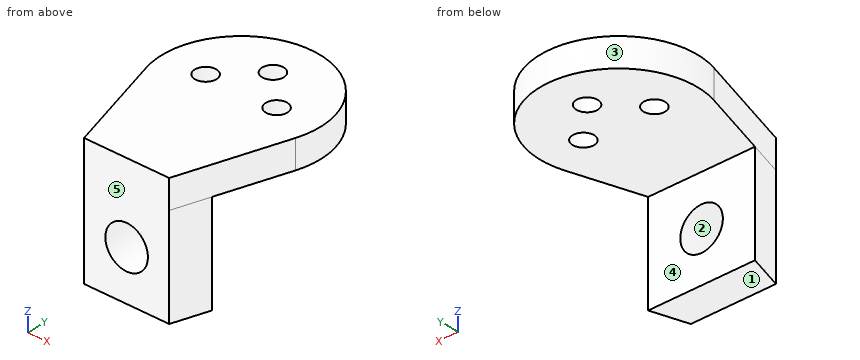
```python
from build123d import *

# Parameters (mm, degrees)
SKETCH1_R           = 55
BOSS_EXTRUDE1_DEPTH = 20
BOSS_EXTRUDE2_DEPTH = 20
CUT_EXTRUDE2_REACH  = 22
SKETCH4_R           = 7.5
BOSS_EXTRUDE3_DEPTH = 70
CUT_EXTRUDE3_REACH  = 27
SKETCH6_R           = 15


with BuildPart() as part:
    # Sketch1 → Boss-Extrude1 (new body)
    with BuildSketch(Plane.XY):
        Circle(SKETCH1_R)
    extrude(amount=BOSS_EXTRUDE1_DEPTH)

    # Sketch2 → Boss-Extrude2 (add)
    with BuildSketch(Plane.XY.offset(20)):
        with BuildLine():
            ThreePointArc((52.597301626, -16.078677236), (0, -55), (-52.597301626, -16.078677236))
            Line((-52.597301626, -16.078677236), (-30, -90))
            Line((-30, -90), (30, -90))
            Line((30, -90), (52.597301626, -16.078677236))
        make_face()
    extrude(amount=-BOSS_EXTRUDE2_DEPTH)

    # Sketch4 → Cut-Extrude2 (cut, up to next)
    with BuildSketch(Plane(origin=(0, 0, 0), x_dir=(-1, 0, 0), z_dir=(0, 0, -1)), mode=Mode.PRIVATE) as cut_extrude2_sk1:
        with Locations((0, 25)):
            Circle(SKETCH4_R)
    cut_extrude2_tool1 = extrude(cut_extrude2_sk1.sketch, amount=-CUT_EXTRUDE2_REACH, mode=Mode.PRIVATE) & part.part
    add(cut_extrude2_tool1.solids().sort_by_distance((0, 25, 0))[0], mode=Mode.SUBTRACT)
    # Sketch4 → Cut-Extrude2 (cut, up to next)
    with BuildSketch(Plane(origin=(0, 0, 0), x_dir=(-1, 0, 0), z_dir=(0, 0, -1)), mode=Mode.PRIVATE) as cut_extrude2_sk2:
        with Locations((-25, 0)):
            Circle(SKETCH4_R)
    cut_extrude2_tool2 = extrude(cut_extrude2_sk2.sketch, amount=-CUT_EXTRUDE2_REACH, mode=Mode.PRIVATE) & part.part
    add(cut_extrude2_tool2.solids().sort_by_distance((25, 0, 0))[0], mode=Mode.SUBTRACT)
    # Sketch4 → Cut-Extrude2 (cut, up to next)
    with BuildSketch(Plane(origin=(0, 0, 0), x_dir=(-1, 0, 0), z_dir=(0, 0, -1)), mode=Mode.PRIVATE) as cut_extrude2_sk3:
        with Locations((25, 0)):
            Circle(SKETCH4_R)
    cut_extrude2_tool3 = extrude(cut_extrude2_sk3.sketch, amount=-CUT_EXTRUDE2_REACH, mode=Mode.PRIVATE) & part.part
    add(cut_extrude2_tool3.solids().sort_by_distance((-25, 0, 0))[0], mode=Mode.SUBTRACT)

    # Sketch5 → Boss-Extrude3 (add)
    with BuildSketch(Plane(origin=(0, 0, 0), x_dir=(-1, 0, 0), z_dir=(0, 0, -1))):
        Polygon((37.642348913, -65), (-37.642348913, -65), (-30, -90), (30, -90), align=None)
    extrude(amount=BOSS_EXTRUDE3_DEPTH)

    # Sketch6 → Cut-Extrude3 (cut, up to next)
    with BuildSketch(Plane(origin=(0, -65, 0), x_dir=(1, 0, 0), z_dir=(0, 1, 0)), mode=Mode.PRIVATE) as cut_extrude3_sk1:
        with Locations((0, 35)):
            Circle(SKETCH6_R)
    cut_extrude3_tool1 = extrude(cut_extrude3_sk1.sketch, amount=-CUT_EXTRUDE3_REACH, mode=Mode.PRIVATE) & part.part
    add(cut_extrude3_tool1.solids().sort_by_distance((0, -65, -35))[0], mode=Mode.SUBTRACT)


solid = part.part
```
CAD build for the part. Positions are in the model's coordinates, mm. Face numbers are marked on the shaded views. A direction names the side the tool comes from. Coordinates: 2 decimals unless noted, no trailing zeros. Order: outer loops, then holes, each group sorted by start corner. A loop starts at its lowest first (then second) coordinate and runs counter-clockwise, first axis right, second up. Notation, with made-up numbers: M 83.5,39.5 L 140.5,39.5 A34 cw 140.5,73.5 Z; hole C 12,21 d2. An arc over 180 degrees is marked long. Answer as CSV lines item,"result".
1) Cut at C-C (x = 0). List the corners of the cut face in (y, z).
Verdict:
outline,"M -90,-70 L -65,-70 L -65,-50 L -90,-50 Z; M -90,-20 L -65,-20 L -65,0 L 17.5,0 L 17.5,20 L -90,20 Z; M 32.5,0 L 55,0 L 55,20 L 32.5,20 Z"
2) Cut at D-D (y = 25). List the corners of the cut face in (x, z).
Verdict:
outline,"M -48.99,0 L -7.5,0 L -7.5,20 L -48.99,20 Z; M 7.5,0 L 48.99,0 L 48.99,20 L 7.5,20 Z"
3) Drill centre lines: L1, parallel to Z at x = 0, y = -72.75; L2, parallel to Z at x = -36, y = 29.5; L3, parallel to Y at x = -29, z = -20.5. Where is each one in solid material? Low to high. Write a range as from..to.
Verdict:
L1,"-70..-50, -20..20"
L2,"0..20"
L3,"-90..-65"
4) Cut at A-A (y = 0). List the corners of the cut face in (x, z).
Verdict:
outline,"M -55,0 L -32.5,0 L -32.5,20 L -55,20 Z; M -17.5,0 L 17.5,0 L 17.5,20 L -17.5,20 Z; M 32.5,0 L 55,0 L 55,20 L 32.5,20 Z"
5) Flat gauge pins, fed straight in: P1, Ø12, axis at x = -25, y = 0, coming from the -Z side; P2, Ø10, axis at x = -42.5, z = -44, coming from the +Y side; P3, Ø17, axis at x = 25, y = 0, coming from the +Z side; P4, Ø17, axis at x = 0, y = 25, coming from the -Z side. Where does each tip first touch, or does it go through?
Verdict:
P1,"through"
P2,"y = -65"
P3,"z = 20"
P4,"z = 0"
6) Mould opens along Z. For the marked faces 1, 2 and 3 say: released by +Z, released by -Z, zero draft, split by the parting line, or undercut.
Verdict:
face 1,"released by -Z"
face 2,"undercut"
face 3,"zero draft"
7) Cut at B-B (z = -35). List the corners of the cut face in (x, y).
Verdict:
outline,"M -37.64,-65 L -30,-90 L -15,-90 L -15,-65 Z; M 15,-90 L 30,-90 L 37.64,-65 L 15,-65 Z"
8) 3-axis set-ups, long thin cutter, end or side, ignore diameter. For the marked faces 4 and 5: which of +Z, -Z, +X, -X, +Y, -Y reach the whole face in a straight line?
Verdict:
face 4,"-Z, +X, -X, +Y"
face 5,"+Z, -Z, +X, -X, -Y"
